Part print with two shaded views. Sizes in mm from the minimum x, y, z corner. Round coordinates to 2 decimals unless told otherwise and drop trailing zeros. Loops run counter-clockwise (first coordinate to the right, second up) from the corner with the lowest first, then second, coordinate; pieces in that order, holes last. Notation, with made-up numbers: (-31, 17.25) - (-23, 17.25) arc R10 cw to (-23, 30.25) - close; hole circle Ø2 at (22, 50.25). An arc over 180 degrees is marked (long way). Write each question's results on one line, items separated by ' | '. Start each with the question number.
(1) Drill centre lines: L1, parallel to Z at x = 110, y = 1.4; L2, parallel to Y at x = 176, z = 158; L3, parallel to X at y = 12.5, z = 138. Where is each one in solid material? Low to high.
(2) Cut at D-D, the plane z = 68. List the corners of the cut face in (x, y), then the cut area to 3 significant figures.
(3) Flat gauge pins, fed straight in: P1, Ø10, axis at x = 84, z = 187, coming from the +Y side; P2, Ø5, axis at x = 140, y = 13, coming from the +Z side; P3, Ø2, axis at y = 17, z = 76, coming from the +X side. Where does each tip first touch, or does it go through?
(4) Cut at A-A, the plane y = 10.25. List the corners of the cut face in (x, z).
(5) Mould opens along Z. For the marked faces 1 and 2 say: released by +Z, released by -Z, zero draft, split by the parting line, or undercut.
(6) Cut at B-B, the plane z = 113.5. List the corners of the cut face in (x, y), then the cut area to 3 significant figures.
(7) Cut at C-C, the plane x = 152. List the corners of the cut face in (y, z), then the cut area to 3 significant figures.
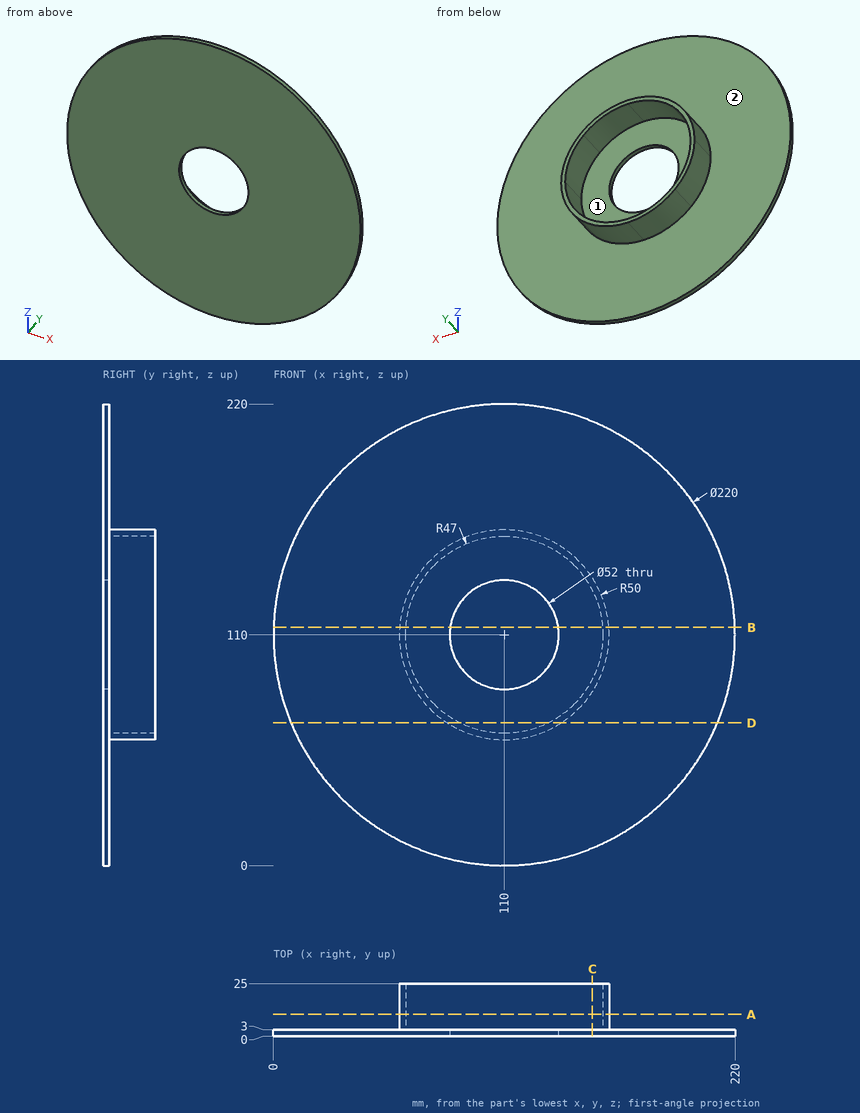
A:
1) L1: 0 to 84, 136 to 220 | L2: 0 to 3 | L3: 68.58 to 72.25, 147.75 to 151.42
2) outline: (8.33, 0) - (211.67, 0) - (211.67, 3) - (137.13, 3) - (137.13, 25) - (131.1, 25) - (131.1, 3) - (88.9, 3) - (88.9, 25) - (82.87, 25) - (82.87, 3) - (8.33, 3) - close | area: 876 mm2
3) P1: y = 3 | P2: z = 151.76 | P3: x = 147.56
4) outline: circle Ø100 at (110, 110); hole circle Ø94 at (110, 110)
5) face 1: undercut | face 2: zero draft
6) outline: (0.06, 0) - (84.24, 0) - (84.24, 3) - (63.13, 3) - (63.13, 25) - (60.12, 25) - (60.12, 3) - (0.06, 3) - close; (135.76, 0) - (219.94, 0) - (219.94, 3) - (159.88, 3) - (159.88, 25) - (156.87, 25) - (156.87, 3) - (135.76, 3) - close | area: 637 mm2
7) outline: (0, 8.33) - (3, 8.33) - (3, 82.87) - (25, 82.87) - (25, 88.9) - (3, 88.9) - (3, 131.1) - (25, 131.1) - (25, 137.13) - (3, 137.13) - (3, 211.67) - (0, 211.67) - close | area: 876 mm2
